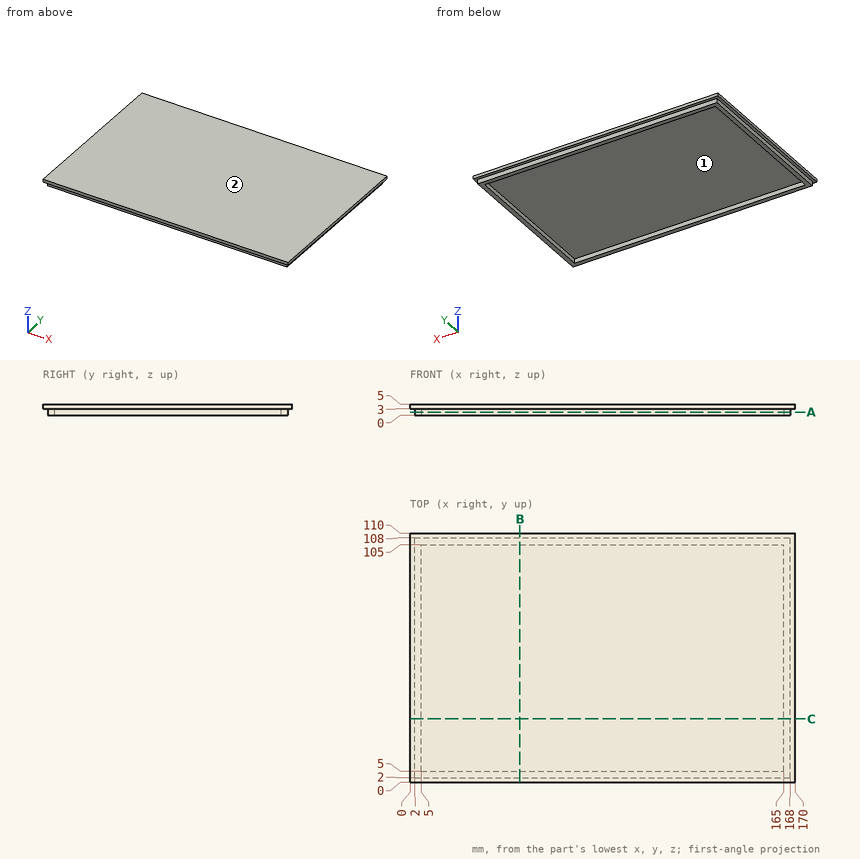
Source: three-view drawing plus pictorial views. Frame: mm from the lowest corner of the part. A direction names the side the tool comes from. Round coordinates to 2 decimals unless told otherwise and drop trailing zeros. Write each loop counter-clockwise with the first axis right and the second up, starting at its lowest first coordinate (ties: lowest second). Pieces come first, ordered by that corner, then holes. Notation, with made-up numbers: M 88.5,15 L 134.5,15 A17 ccw 134.5,30 Z; hole C -3.5,-4 d8. An arc over 180 degrees is marked long. Use CSV: the item, a comma, the result in double quotes. Start each with the question number.
Q1. Access query for the marked faces 1 and 2. Directions: +Z, -Z, +X, -X, +Y, -Y. A direction counts if a zero-diameter tool reaches every point of the face in a straight line with its end or side. Return the directions, or none.
Q2. Line query: line 1 (Y direction, x = 77, z = 1.85); line 2 (X direction, y = 30.5, z = 0.75); line 3 (Z direction, x = 54.5, y = 78). Output: solid intervals per line, ascending. Write a range as from..to.
Q3. Cut plane C-C on y = 28. Output: boundary loops of the cut face in (x, z), plus the area to 3 significant figures.
Q4. Cut plane A-A on z = 1.4. Output: boundary loops of the cut face in (x, y).
Q5. First-contact query: P1, Ø0.9, axis at y = 68.5, z = 1.5, coming from the -X side; P2, Ø2, axis at x = 77.5, y = 96, coming from the -Z side; P3, Ø1.5, axis at x = 107, z = 1, coming from the -Y side. Flat tips, straight axial feed; report the tip coordinate or a pass-through.
Q6. Cut plane B-B on x = 48.5. Output: boundary loops of the cut face in (y, z), plus the area to 3 significant figures.
Results found:
1,face 1,"-Z"
1,face 2,"+Z, +X, -X, +Y, -Y"
2,line 1,"2..5, 105..108"
2,line 2,"2..5, 165..168"
2,line 3,"3..5"
3,outline,"M 0,3 L 2,3 L 2,0 L 5,0 L 5,3 L 165,3 L 165,0 L 168,0 L 168,3 L 170,3 L 170,5 L 0,5 Z"
3,area,"358 mm^2"
4,outline,"M 2,2 L 168,2 L 168,108 L 2,108 Z; hole M 5,5 L 165,5 L 165,105 L 5,105 Z"
5,P1,"x = 2"
5,P2,"z = 3"
5,P3,"y = 2"
6,outline,"M 0,3 L 2,3 L 2,0 L 5,0 L 5,3 L 105,3 L 105,0 L 108,0 L 108,3 L 110,3 L 110,5 L 0,5 Z"
6,area,"238 mm^2"
